```python
from build123d import *

# Parameters (mm, degrees)
SKETCH025_W     = 25
SKETCH025_H     = 20
SKETCH025_R     = 2.5
PAD013_DEPTH    = 4
SKETCH026_W     = 10
SKETCH026_H     = 20
PAD014_DEPTH    = 10
SKETCH027_R     = 4
POCKET013_DEPTH = 20.001


with BuildPart() as part:
    # Sketch025 → Pad013 (new body)
    with BuildSketch(Plane.XZ):
        Rectangle(SKETCH025_W, SKETCH025_H)
        with Locations((-8.5, 0)):
            Circle(SKETCH025_R, mode=Mode.SUBTRACT)
        with Locations((8.5, 0)):
            Circle(SKETCH025_R, mode=Mode.SUBTRACT)
    extrude(amount=PAD013_DEPTH)

    # Sketch026 (on Face7 of Pad013) → Pad014 (join)
    with BuildSketch(Plane(origin=(0, 0, 0), x_dir=(1, 0, 0), z_dir=(0, 1, 0))):
        Rectangle(SKETCH026_W, SKETCH026_H)
    extrude(amount=PAD014_DEPTH)

    # Sketch027 (on Face5 of Pad014) → Pocket013 (cut, through all)
    with BuildSketch(Plane(origin=(0, 0, 10), x_dir=(-1, 0, 0), z_dir=(0, 0, 1))):
        with Locations((0, -5)):
            Circle(SKETCH027_R)
    extrude(amount=-POCKET013_DEPTH, mode=Mode.SUBTRACT)


solid = part.part
```
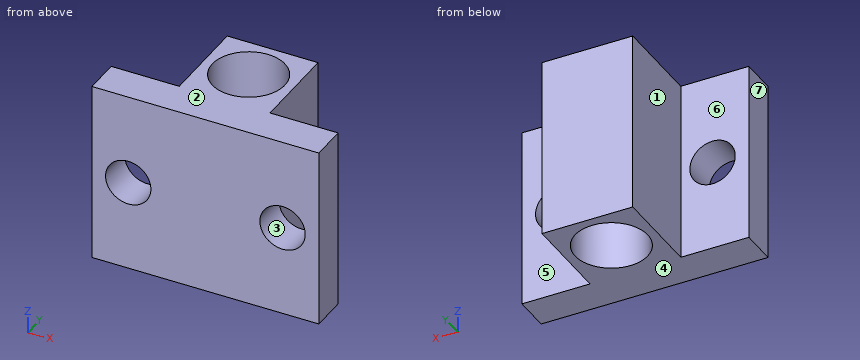
Model file for the job. Use its own axes, mm. Face numbers are marked on the shaded views. A direction names the side the tool comes from. Coordinates: 2 decimals unless noted, no trailing zeros. Loops run counter-clockwise (first coordinate to the right, second up) from the corner with the lowest first, then second, coordinate; pieces in that order, holes last. Notation, with made-up numbers: (38, 34) - (68, 34) arc R22 cw to (68, 56) - close; hole circle Ø10 at (-24, 50). An arc over 180 degrees is marked (long way). Answer as a JSON object with one key per item and string values. Group by question number.
(1) Flat gauge pins, fed straight in: pin 1 (3 mm diameter, centred on x = -8.5, z = -2.5, fed in from +Y); pin 2 (5 mm diameter, centred on y = 7.5, z = 0, fed in from +X); pin 3 (3 mm diameter, centred on y = 7.5, z = -0.5, fed in from -X). Where does each tip first touch, or does it go through?
(2) Cut at D-D (y = -3). Give the cut face in (x, z).
(3) Two-plate mould, pull along Z, no slides. Class the marked faces 1, 2, 3 and 4: released by +Z, released by -Z, zero draft, split by the parting line, or undercut.
(4) Cut at B-B (x = 7). Give the cut face in (y, z).
(5) Cut at A-A (z = 0). Give the cut face in (x, y).
(6) Tool access for the marked faces 5, 6 and 7: list every direction of +Z, -Z, +X, -X, +Y, -Y with a clear straight run to the whole face (end or side of a thin tool).
(7) Probe line 1 along X through (y, z) = (5, 2.25); line 2 along Z through (x, y) = (8.5, -2.2); line 3 along Y through (x, z) = (0, -5.75). List the from-to ranges inside material, lowest first.
(8) Cut at C-C (y = 5). Give the cut face in (x, z).
Geometry says:
{
 "1": {"pin 1": "stops at y = 0", "pin 2": "stops at x = 5", "pin 3": "stops at x = -5"},
 "2": {"outline": "(-12.5, -10) - (12.5, -10) - (12.5, 10) - (-12.5, 10) - close; hole circle Ø5 at (-8.5, 0); hole circle Ø5 at (8.5, 0)"},
 "3": {"face 1": "zero draft", "face 2": "released by +Z", "face 3": "undercut", "face 4": "released by -Z"},
 "4": {"outline": "(-4, -10) - (0, -10) - (0, -2) - (-4, -2) - close; (-4, 2) - (0, 2) - (0, 10) - (-4, 10) - close"},
 "5": {"outline": "(-12.5, -4) - (-11, -4) - (-11, 0) - (-12.5, 0) - close; (-6, -4) - (6, -4) - (6, 0) - (5, 0) - (5, 10) - (-5, 10) - (-5, 0) - (-6, 0) - close; (11, -4) - (12.5, -4) - (12.5, 0) - (11, 0) - close; hole circle Ø8 at (0, 5)"},
 "6": {"face 5": "+Z, -Z, +X, +Y", "face 6": "+Z, -Z, -X, +Y", "face 7": "+Z, -Z, -X, +Y, -Y"},
 "7": {"line 1": "x = -5 to -4, 4 to 5", "line 2": "z = -10 to -2.5, 2.5 to 10", "line 3": "y = -4 to 1, 9 to 10"},
 "8": {"outline": "(-5, -10) - (-4, -10) - (-4, 10) - (-5, 10) - close; (4, -10) - (5, -10) - (5, 10) - (4, 10) - close"}
}
